Input: part model. Units: mm. Frame: model coordinates. Face numbers are marked on the shaded views. A direction names the side the tool comes from. Coordinates: 2 decimals unless noted, no trailing zeros. Loops run counter-clockwise (first coordinate to the right, second up) from the corner with the lowest first, then second, coordinate; pieces in that order, holes last. Notation, with made-up numbers: (-4, -34.5) - (3, -34.5) arc R31 cw to (3, -2.5) - close; hole circle Ø6 at (-32, 62.5). An arc over 180 degrees is marked (long way). Write item = value, one per line. Start each with the question number.
Autodesk Inventor part; units mm, degrees
ref_plane "YZ Plane" through (0, 0, 0) normal (1, 0, 0) x (0, 1, 0)
ref_plane "XZ Plane" through (0, 0, 0) normal (0, 1, 0) x (-1, 0, 0)
ref_plane "XY Plane" through (0, 0, 0) normal (0, 0, 1) x (1, 0, 0)
sketch "Sketch2" plane through (0, 0, 0) normal (0, 0, 1) x (1, 0, 0)
  arc A0 (3.57, -3.175) -> (3.57, 3.175) centre (3.57, 0) ccw
  arc A1 (0, 3.175) -> (0, -3.175) centre (0, 0) ccw
  line L0 (0, 3.175) -> (3.57, 3.175)
  line L1 (0, -3.175) -> (3.57, -3.175)
  dimension "d14" = 6.35
  dimension "d15" = 6.35
  dimension "d16" = 0
  dimension "d17" = 0
  dimension "d18" = 3.57
  dimension "d19" = 0
extrude "Extrusion2" add sketch "Sketch2" along normal blind 8.509
sketch "Sketch3" plane through (0, 0, 8.509) normal (0, 0, 1) x (1, 0, 0)
  point P0 (0, 0)
  point P1 (3.57, 0)
  dimension "d22" = 3.57
  dimension "d23" = 0
hole "Hole1" at (3.57, 0, 8.509) direction (0, 0, -1) diameter 2.459 depth 3.81 tip angle 118
sketch "Sketch4" plane through (0, 0, 0) normal (0, 0, -1) x (-1, 0, 0)
  point P0 (0, 0)
hole "Hole2" at (0, 0, 0) direction (0, 0, 1) diameter 2.459 depth 3.81 tip angle 118
sketch "Sketch5" plane through (0, 0, 0) normal (0, 0, -1) x (-1, 0, 0)
  arc A0 (-3.57, 3.175) -> (-3.57, -3.175) centre (-3.57, 0) ccw
  arc A1 (0, 3.175) -> (0, -3.175) centre (0, 0) ccw
  line L0 (0, 3.175) -> (-3.57, 3.175)
  arc A2 (0, -3.175) -> (0, 3.175) centre (0, 0) ccw
  line L1 (0, -3.175) -> (-3.57, -3.175)
  dimension "d42" = 3.57
extrude "Extrusion3" cut sketch "Sketch5" against normal blind 3.175 from surface at 0 contours L0 A1 L1 A0
sketch "Sketch6" plane through (0, 0, 8.509) normal (0, 0, 1) x (1, 0, 0)
  arc A0 (3.5699, 3.1751) -> (3.5474, -3.175) centre (3.57, 0) ccw
  line L0 (3.5699, 3.1751) -> (-0.0001, 3.175)
  line L1 (0, -3.175) -> (3.57, -3.175)
  line L2 (3.5474, -3.175) -> (0, -3.175)
  arc A1 (-0.0001, 3.175) -> (0, -3.175) centre (0, 0) ccw
  dimension "d43" = 3.57
extrude "Extrusion4" cut sketch "Sketch6" against normal blind 3.175
properties part number "PC104_EM-113 standoff_3.57"
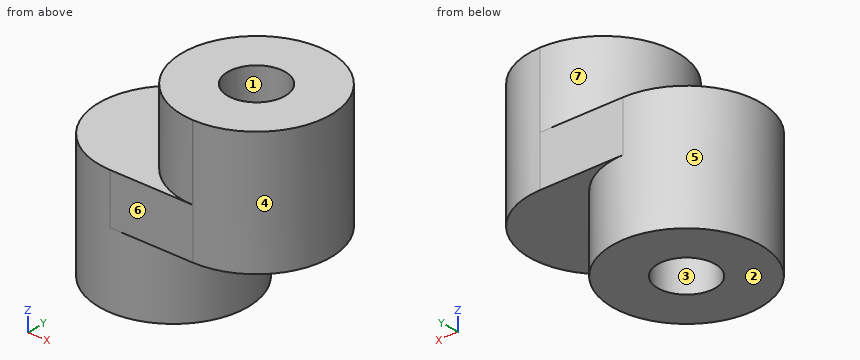
Item 1: Cut plane C-C on x = 5.5. Return loops of the section in (y, z) (3 decimals), plus the area to 3 significant figures.
Item 2: Cut plane A-A on y = -2.5. Return loops of the section in (x, z) (3 decimals).
Item 3: Pull-direction query (X, two-part tool) for the marked faces 1, 2, 3 and 4; classes: pulls with the +X half, pulls with the -X half, needs draft (parallel to the pull), parting line crosses it, or undercut.
Item 4: Ray query, line 1 (Y direction, x = 0, z = 2.6) (1 decimal); line 2 (X direction, y = 0, z = 7.25) (1 decimal). Return the intervals inside material, ascending.
Item 5: Access query for the marked faces 5, 6 and 7. Directions: +Z, -Z, +X, -X, +Y, -Y. A direction counts if a zero-diameter tool reaches every point of the face in a straight line with its end or side. Return the directions, or none.
Item 6: Pin query (flat end, axial travel): pin 1 (1.5 mm diameter, centred on y = -0.5, z = 2.5, fed in from +X); pin 2 (3 mm diameter, centred on x = 5, y = 1.5, fed in from -Z) (3 decimals); pin 3 (2 mm diameter, centred on y = -2.5, z = 7, fed in from +X). Return the tip coordinate at first contact, or that it passes through.
Recorded:
q1.outline = (-2.521, 3.175) - (2.521, 3.175) - (2.521, 8.509) - (-2.521, 8.509) - close
q1.area = 26.9 mm²
q2.outline = (-1.957, 0) - (1.957, 0) - (1.957, 3.175) - (5.527, 3.175) - (5.527, 8.509) - (1.613, 8.509) - (1.613, 5.334) - (-1.957, 5.334) - close
q3.face_1 = undercut
q3.face_2 = needs draft
q3.face_3 = undercut
q3.face_4 = pulls with the +X half
q4.line_1 = -3.2 to -1.2, 1.2 to 3.2
q4.line_2 = 0.4 to 2.3, 4.8 to 6.7
q5.face_5 = -Z
q5.face_6 = +Z, -Z, +X, -X, -Y
q5.face_7 = +Z, -X
q6.pin_1 = 6.74
q6.pin_2 = 3.175
q6.pin_3 = 6.37
